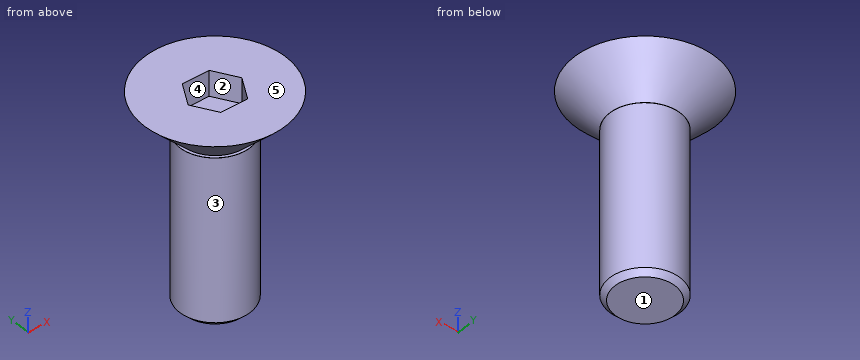
Solid Edge part; units mm, degrees
sketch "Sketch1" plane through (0, 0, 0) normal (0, 0, 1) x (1, 0, 0)
  circle A0 centre (0, 0) radius 12
extrude "Protrusion1" add sketch "Sketch1" along normal blind 6.5
sketch "Sketch2" plane through (0, 0, 0) normal (0, 0, -1) x (1, 0, 0)
  circle A0 centre (0, 0) radius 6
extrude "Protrusion2" add sketch "Sketch2" along normal blind 28.5
sketch "Sketch3" plane through (0, 0, -28.5) normal (0, 0, -1) x (1, 0, 0)
  circle A0 centre (0, 0) radius 5.9997
extrude "Cutout1" cut sketch "Sketch3" against normal blind 28.4715 flip side to cut
chamfer "Chamfer_1" distance 0.9 angle 45 1 edges at (-5.9997, 0, -28.5)
sketch "Sketch4" plane through (0, 0, 6.5) normal (0, 0, 1) x (1, 0, 0)
  line L0 (-2.3094, 4) -> (2.3094, 4)
  line L1 (4.6188, 0) -> (2.3094, 4)
  line L2 (2.3094, -4) -> (4.6188, 0)
  line L3 (-2.3094, -4) -> (2.3094, -4)
  line L4 (-4.6188, 0) -> (-2.3094, -4)
  line L5 (-2.3094, 4) -> (-4.6188, 0)
extrude "Cutout2" cut sketch "Sketch4" against normal blind 4.3333
sketch "Sketch5" plane through (0, 0, 0) normal (0, -1, 0) x (1, 0, 0)
  line L0 (12, 6.5) -> (5.5, 0)
  line L1 (5.5, 0) -> (12, 0)
  line L2 (12, 0) -> (12, 6.5)
revolve "RevolvedCutout1" cut sketch "Sketch5" angle 360 about axis through (0, 0, 14.0017) along (0, 0, -1)
properties part number "24104732"
Input: part model. Units: mm. Frame: model coordinates. Face numbers are marked on the shaded views. A direction names the side the tool comes from. Coordinates: 2 decimals unless noted, no trailing zeros. Loops run counter-clockwise (first coordinate to the right, second up) from the corner with the lowest first, then second, coordinate; pieces in that order, holes last.
(1) First-contact query: pin 1 Ø5 at (y, z) = (-6, -14) entering from -X; pin 2 Ø6 at (x, z) = (1, -23) entering from +Y; pin 3 Ø10 at (y, z) = (5.5, -19.5) entering from -X. Flat tips, straight axial feed; report the tip coordinate or a pass-through.
(2) Material intervals for probe 1 along Z at (x, y) = (2.75, 3); probe 2 along Y at (x, z) = (-4.25, -3); probe 3 along Y at (x, z) = (-4.75, -12), sorted ascending.
(3) Pull-direction query (X, two-part tool) for the marked faces 3, 4 and 5; classes: released by +X, released by -X, zero draft, split by the parting line, or undercut.
(4) Set-up query: the marked faces 1 and 2. Return all of +Z, -Z, +X, -X, +Y, -Y with unobstructed straight access to the full face (end or side cutting, diameter ignored); none if empty.
(5) Section B-B on z = -4. Return the cut outline in (x, y), then the cut area to 3 significant figures.
Data:
1. pin 1: stops at x = -4.87
1. pin 2: stops at y = 6
1. pin 3: stops at x = -5.98
2. probe 1: z = -28.5 to 2.17
2. probe 2: y = -4.23 to 4.23
2. probe 3: y = -3.67 to 3.67
3. face 3: split by the parting line
3. face 4: undercut
3. face 5: zero draft
4. face 1: -Z, +X, -X, +Y, -Y
4. face 2: +Z
5. outline: circle Ø12 at (0, 0)
5. area: 113 mm2
